Build history of the part. All positions in model axes, mm. Face numbers are marked on the shaded views. A direction names the side the tool comes from. Round coordinates to 2 decimals unless told otherwise and drop trailing zeros. Write each loop counter-clockwise with the first axis right and the second up, starting at its lowest first coordinate (ties: lowest second). Pieces come first, ordered by that corner, then holes. Notation, with made-up numbers: (-29, 83.5) -> (-1, 83.5) arc R23 cw to (-1, 109.5) -> close; hole circle Ø8 at (80.5, 4). An arc over 180 degrees is marked (long way). Answer in a Markdown table with one row per item. Add a question column.
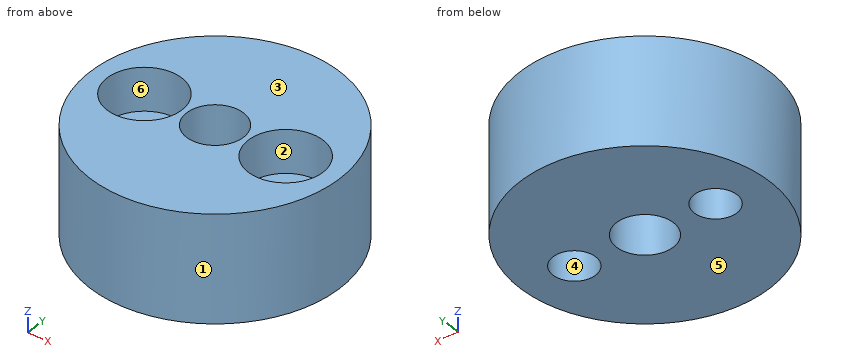
Autodesk Inventor part; units mm, degrees
ref_plane "YZ Plane" through (0, 0, 0) normal (1, 0, 0) x (0, 1, 0)
ref_plane "XZ Plane" through (0, 0, 0) normal (0, 1, 0) x (-1, 0, 0)
ref_plane "XY Plane" through (0, 0, 0) normal (0, 0, 1) x (1, 0, 0)
sketch "Sketch1" plane through (0, 0, 0) normal (0, 0, 1) x (1, 0, 0)
  circle A0 centre (0, 0) radius 17.5
  circle A1 centre (0, 0) radius 4
  line L0 (-10, 0) -> (10, 0) construction
  circle A2 centre (-10, 0) radius 3
  circle A3 centre (10, 0) radius 3
  dimension "d0" = 35
  dimension "d1" = 8
  dimension "d7" = 20
  dimension "d8" = 6
extrude "Extrusion1" add sketch "Sketch1" along normal blind 15
sketch "Sketch3" plane through (0, 0, 15) normal (0, 0, 1) x (1, 0, 0)
  circle A0 centre (10, 0) radius 3
  circle A1 centre (-10, 0) radius 3
  circle A2 centre (-10, 0) radius 5.25
  circle A3 centre (10, 0) radius 5.25
  dimension "d9" = 10.5
extrude "Extrusion3" cut sketch "Sketch3" against normal blind 6
properties part number "gear thrust cup"
(1) Saw through at A-A (x = 0). List the corners of the cut face in (y, z).
(2) Which spindle directions (+Z, -Z, +X, -X, +Y, -Y) get a long thin tool onto all of the face, cutting with end or side? Do the marked faces 5 and 6. Say none if no direction does.
(3) Saw through at B-B (y = 0). List the corners of the cut face in (x, z), plus the area to 3 significant figures.
(4) Probe line 1 along Y through (x, z) = (0, 8); line 2 along Y through (x, z) = (10, 12.3); line 3 along Y through (x, z) = (15.5, 13.75). List the from-to ranges inside material, lowest first.
(5) Saw through at D-D (x = 10). List the corners of the cut face in (y, z).
(6) Drop flat-ended pins along their axis: P1, Ø3.5, axis at x = -10, y = 0, coming from the +Z side; P2, Ø3, axis at x = 12, y = -0.5, coming from the +Z side; P3, Ø6, axis at x = 11, z = 2, coming from the -Y side; P4, Ø5, axis at x = 4, z = 9.5, coming from the +Y side. Give the stop position or say it passes through.
(7) Mould opens along Y. For the marked faces 1, 2, 3 and 4 say: pulls with the +Y half, pulls with the -Y half, needs draft (parallel to the pull), parting line crosses it, or undercut.
(8) Saw through at C-C (z = 12.5). List the corners of the cut face in (x, y), plus the area to 3 significant figures.
Answer sheet:
| question | item | result |
|---|---|---|
| 1 | outline | (-17.5, 0) -> (-4, 0) -> (-4, 15) -> (-17.5, 15) -> close; (4, 0) -> (17.5, 0) -> (17.5, 15) -> (4, 15) -> close |
| 2 | face 5 | -Z, +X, -X, +Y, -Y |
| 2 | face 6 | +Z |
| 3 | outline | (-17.5, 0) -> (-13, 0) -> (-13, 9) -> (-15.25, 9) -> (-15.25, 15) -> (-17.5, 15) -> close; (-7, 0) -> (-4, 0) -> (-4, 15) -> (-4.75, 15) -> (-4.75, 9) -> (-7, 9) -> close; (4, 0) -> (7, 0) -> (7, 9) -> (4.75, 9) -> (4.75, 15) -> (4, 15) -> close; (13, 0) -> (17.5, 0) -> (17.5, 15) -> (15.25, 15) -> (15.25, 9) -> (13, 9) -> close |
| 3 | area | 171 mm² |
| 4 | line 1 | y = -17.5 to -4, 4 to 17.5 |
| 4 | line 2 | y = -14.36 to -5.25, 5.25 to 14.36 |
| 4 | line 3 | y = -8.12 to 8.12 |
| 5 | outline | (-14.36, 0) -> (-3, 0) -> (-3, 9) -> (-5.25, 9) -> (-5.25, 15) -> (-14.36, 15) -> close; (3, 0) -> (14.36, 0) -> (14.36, 15) -> (5.25, 15) -> (5.25, 9) -> (3, 9) -> close |
| 6 | P1 | passes through |
| 6 | P2 | stops at z = 9 |
| 6 | P3 | stops at y = -15.56 |
| 6 | P4 | stops at y = 17.44 |
| 7 | face 1 | parting line crosses it |
| 7 | face 2 | undercut |
| 7 | face 3 | needs draft |
| 7 | face 4 | undercut |
| 8 | outline | circle Ø35 at (0, 0); hole circle Ø10.5 at (-10, 0); hole circle Ø8 at (0, 0); hole circle Ø10.5 at (10, 0) |
| 8 | area | 739 mm² |
